```python
from build123d import *

# Parameters (mm, degrees)
IZIM1_R                     = 12.5
Y_KSEKLIK_EKSTR_ZYON1_DEPTH = 546
IZIM2_R                     = 4.25
KES_EKSTR_ZYON1_DEPTH       = 20
KES_EKSTR_ZYON2_START       = -20
IZIM3_R                     = 4.25
KES_EKSTR_ZYON2_DEPTH       = 20
KES_EKSTR_ZYON3_START       = -36
IZIM4_R                     = 12.5
IZIM4_R_2                   = 10
KES_EKSTR_ZYON3_DEPTH       = 36
IZIM5_R                     = 12.5
IZIM5_R_2                   = 10
KES_EKSTR_ZYON4_DEPTH       = 36
IZIM8_W                     = 3.7
IZIM8_H                     = 1.2
RADYUS1_R                   = 1


with BuildPart() as part:
    # Çizim1 → Yükseklik-Ekstrüzyon1 (new body)
    with BuildSketch(Plane.XY):
        Circle(IZIM1_R)
    extrude(amount=Y_KSEKLIK_EKSTR_ZYON1_DEPTH)

    # Çizim2 → Kes-Ekstrüzyon1 (cut)
    with BuildSketch(Plane.XY.offset(546)):
        Circle(IZIM2_R)
    extrude(amount=-KES_EKSTR_ZYON1_DEPTH, mode=Mode.SUBTRACT)

    # Çizim3 → Kes-Ekstrüzyon2 (cut)
    with BuildSketch(Plane(origin=(0, 0, 0), x_dir=(-1, 0, 0), z_dir=(0, 0, -1)).offset(KES_EKSTR_ZYON2_START)):
        with Locations(Location((0, 0, 0), (0, 0, 180))):
            Circle(IZIM3_R)
    extrude(amount=KES_EKSTR_ZYON2_DEPTH, mode=Mode.SUBTRACT)

    # Çizim4 → Kes-Ekstrüzyon3 (cut)
    with BuildSketch(Plane.XY.offset(546).offset(KES_EKSTR_ZYON3_START)):
        Circle(IZIM4_R)
        Circle(IZIM4_R_2, mode=Mode.SUBTRACT)
    extrude(amount=KES_EKSTR_ZYON3_DEPTH, mode=Mode.SUBTRACT)

    # Çizim5 → Kes-Ekstrüzyon4 (cut)
    with BuildSketch(Plane(origin=(0, 0, 0), x_dir=(-1, 0, 0), z_dir=(0, 0, -1))):
        Circle(IZIM5_R)
        with Locations(Location((0, 0, 0), (0, 0, 180))):
            Circle(IZIM5_R_2, mode=Mode.SUBTRACT)
    extrude(amount=-KES_EKSTR_ZYON4_DEPTH, mode=Mode.SUBTRACT)

    # Çizim8 → Kes-Döndür1 (revolve, cut)
    with BuildSketch(Plane(origin=(0, 0, 0), x_dir=(1, 0, 0), z_dir=(0, 1, 0))):
        with Locations((-10, -14)):
            Rectangle(IZIM8_W, IZIM8_H)
        with Locations((-10, -532)):
            Rectangle(IZIM8_W, IZIM8_H)
    revolve(axis=Axis((0, 0, 0), (0, 0, 1)), mode=Mode.SUBTRACT)

    # Radyus1
    radyus1_edges = [part.edges().sort_by_distance(p)[0] for p in [
        (-12.5, 0, 510),
        (-10, 0, 546),
        (-12.5, 0, 36),
        (-10, 0, 0),
    ]]
    fillet(radyus1_edges, radius=RADYUS1_R)


solid = part.part
```
Geometry check sheet. Reference: the model listing, model coordinates, mm. A direction names the side the tool comes from. Give positions to 0.01 mm unless a question says otherwise; leave off trailing zeros. Write each loop counter-clockwise with the first axis right and the second up, starting at its lowest first coordinate (ties: lowest second). Pieces come first, ordered by that corner, then holes.
1) Access from +Z, -Z, +X, -X, +Y, -Y to the whole of each face (thin tool, end or side, straight path). Record for faces 1 (the flat face through (3.8, 7.4, 13.4)), 2 (the cylindrical face through (11.923, 3.755, 269.696)), 3 (the cylindrical face through (-2.17, -9.76, 520.55)), 4 (the flat face through (4, -2, 0)), 5 (the flat face through (9, 5, 36)).
2) Material ranges on L1, parallel to Z at x = -7.75, y = -3; L2, parallel to Y at x = 0, z = 10.75; L3, parallel to Z at x = 1.25, y = 11, recorded low to high.
3) Gauge pin test, flat ends, axial feed: pin 1 (6 mm diameter, centred on x = -5.5, z = 226.5, fed in from +Y); pin 2 (2 mm diameter, centred on y = -4.5, z = 308.5, fed in from -X); pin 3 (1.5 mm diameter, centred on y = 9.5, z = 428, fed in from +X). Record the tip position at first contact, or that the pin passes through.
4) Release check for a two-part mould opening along X. For faces 6 (the flat face through (4, -2, 546)), 7 (the cylindrical face through (-10, 0, 25)), 8 (the flat face through (0, 0, 526)) record: pulls with the +X half, pulls with the -X half, needs draft (parallel to the pull), parting line crosses it, or undercut.
5) Section check A-A, the plane z = 57. Record the boundary of the cut face in (x, y).
Computed:
1. face 1: none
1. face 2: +Z, -Z
1. face 3: +Z
1. face 4: -Z, +X, -X, +Y, -Y
1. face 5: -Z
2. L1: z = 0 to 13.4, 14.6 to 531.4, 532.6 to 546
2. L2: y = -10 to -4.25, 4.25 to 10
2. L3: z = 36 to 510
3. pin 1: stops at y = 12.25
3. pin 2: stops at x = -12
3. pin 3: stops at x = 8.93
4. face 6: needs draft
4. face 7: parting line crosses it
4. face 8: undercut
5. outline: circle Ø25 at (0, 0)
